```python
from build123d import *

# Parameters (mm, degrees)
SKETCH2_W           = 32
SKETCH2_H           = 30
SKETCH2_R           = 1.25
SKETCH2_R_2         = 7.25
BOSS_EXTRUDE1_DEPTH = 2
SKETCH2_4_W         = 32
SKETCH2_4_H         = 2
BOSS_EXTRUDE2_DEPTH = 35
BOSS_EXTRUDE3_DEPTH = 2
FILLET1_R           = 2
SKETCH5_W           = 7
SKETCH5_H           = 25
SKETCH5_R           = 1.6
BOSS_EXTRUDE4_DEPTH = 2
FILLET2_R           = 2
SKETCH14_W          = 16
SKETCH14_H          = 19
CUT_EXTRUDE1_DEPTH  = 52.51698749
CUT_EXTRUDE2_DEPTH  = 56.090834083
EXTRUDE_THIN1_DEPTH = 2
FILLET3_R           = 1
FILLET4_R           = 0.5
SKETCH21_R          = 1.5
CUT_EXTRUDE3_DEPTH  = 10


with BuildPart() as part:
    # Sketch2 → Boss-Extrude1 (new body)
    with BuildSketch(Plane.XY):
        Rectangle(SKETCH2_W, SKETCH2_H)
        with Locations((-8.227241336, 4.75)):
            Circle(SKETCH2_R, mode=Mode.SUBTRACT)
        with Locations((8.227241336, 4.75)):
            Circle(SKETCH2_R, mode=Mode.SUBTRACT)
        with Locations((0, -9.5)):
            Circle(SKETCH2_R, mode=Mode.SUBTRACT)
        Circle(SKETCH2_R_2, mode=Mode.SUBTRACT)
    extrude(amount=BOSS_EXTRUDE1_DEPTH)

    # Sketch2<4> → Boss-Extrude2 (add)
    with BuildSketch(Plane.XY):
        with Locations((0, -16)):
            Rectangle(SKETCH2_4_W, SKETCH2_4_H)
    extrude(amount=BOSS_EXTRUDE2_DEPTH)

    # Sketch3 → Boss-Extrude3 (add)
    with BuildSketch(Plane(origin=(16, 0, 0), x_dir=(0, 0, -1), z_dir=(1, 0, 0))):
        Polygon((-2, 6.21520857), (-22.300940927, -15), (-2, -15), align=None)
    boss_extrude3 = extrude(amount=-BOSS_EXTRUDE3_DEPTH)

    # Mirror1: Boss-Extrude3 across plane
    add(boss_extrude3.mirror(Plane.ZY))

    # Fillet1
    fillet1_edges = [part.edges().sort_by_distance(p)[0] for p in [
        (-16, 15, 1),
        (16, 15, 1),
    ]]
    fillet(fillet1_edges, radius=FILLET1_R)

    # Sketch5 → Boss-Extrude4 (add)
    # profile 1 of 2: a face of its own
    with BuildSketch(Plane(origin=(0, -15, 0), x_dir=(1, 0, 0), z_dir=(0, 1, 0))):
        with Locations((19.5, -17.5)):
            Rectangle(SKETCH5_W, SKETCH5_H)
        with Locations(Location((19.5, -26.5, 0), (0, 0, 180))):
            Circle(SKETCH5_R, mode=Mode.SUBTRACT)
        with Locations(Location((19.5, -17.5, 0), (0, 0, 180))):
            Circle(SKETCH5_R, mode=Mode.SUBTRACT)
        with Locations(Location((19.5, -8.5, 0), (0, 0, 180))):
            Circle(SKETCH5_R, mode=Mode.SUBTRACT)
    # profile 2 of 2: a face of its own
    with BuildSketch(Plane(origin=(0, -15, 0), x_dir=(1, 0, 0), z_dir=(0, 1, 0))):
        with Locations((-19.5, -17.5)):
            Rectangle(SKETCH5_W, SKETCH5_H)
        with Locations(Location((-19.5, -26.5, 0), (0, 0, 180))):
            Circle(SKETCH5_R, mode=Mode.SUBTRACT)
        with Locations(Location((-19.5, -17.5, 0), (0, 0, 180))):
            Circle(SKETCH5_R, mode=Mode.SUBTRACT)
        with Locations(Location((-19.5, -8.5, 0), (0, 0, 180))):
            Circle(SKETCH5_R, mode=Mode.SUBTRACT)
    extrude(amount=-BOSS_EXTRUDE4_DEPTH)

    # Fillet2
    fillet2_edges = [part.edges().sort_by_distance(p)[0] for p in [
        (-23, -16, 5),
        (-16, -16, 5),
        (-16, -16, 30),
        (16, -16, 35),
        (-16, -16, 35),
        (23, -16, 30),
        (16, -16, 30),
        (16, -16, 5),
        (23, -16, 5),
        (-23, -16, 30),
    ]]
    fillet(fillet2_edges, radius=FILLET2_R)

    # Sketch14 → Cut-Extrude1 (cut, through all)
    with BuildSketch(Plane(origin=(0, -15, 0), x_dir=(1, 0, 0), z_dir=(0, 1, 0))):
        with Locations((0, -19.5)):
            Rectangle(SKETCH14_W, SKETCH14_H)
    extrude(amount=-CUT_EXTRUDE1_DEPTH, mode=Mode.SUBTRACT)

    # Sketch20 → Cut-Extrude2 (cut, through all)
    with BuildSketch(Plane.ZY.offset(16)):
        Polygon((2, -12), (5, -15), (2, -15), align=None)
    extrude(amount=-CUT_EXTRUDE2_DEPTH, mode=Mode.SUBTRACT)

    # Sketch15 → Extrude-Thin1 (add)
    with BuildSketch(Plane(origin=(0, -15, 0), x_dir=(1, 0, 0), z_dir=(0, 1, 0))):
        Polygon((6.852633203, -9.033796381), (-9.147366797, -28.033796381), (-6.852633203, -29.966203619), (9.147366797, -10.966203619), align=None)
        Polygon((-9.147366797, -10.966203619), (6.852633203, -29.966203619), (9.147366797, -28.033796381), (-6.852633203, -9.033796381), align=None)
    extrude(amount=-EXTRUDE_THIN1_DEPTH)

    # Fillet3
    fillet3_edges = [part.edges().sort_by_distance(p)[0] for p in [
        (-6.03898805, -16, 10),
        (6.03898805, -16, 10),
        (-8, -16, 12.32870169),
        (-8, -16, 26.67129831),
        (6.03898805, -16, 29),
        (-6.03898805, -16, 29),
        (8, -16, 26.67129831),
        (8, -16, 12.32870169),
        (1.96101195, -16, 19.5),
        (0, -16, 21.82870169),
        (-1.96101195, -16, 19.5),
        (0, -16, 17.17129831),
    ]]
    fillet(fillet3_edges, radius=FILLET3_R)

    # Fillet4
    fillet4_edges = [part.edges().sort_by_distance(p)[0] for p in [
        (15, -12, 2),
        (15, -15, 5),
        (-15, -15, 5),
        (-15, -12, 2),
        (15, 6.21520857, 2),
        (15, -15, 22.300940927),
        (-15, 6.21520857, 2),
        (-15, -15, 22.300940927),
    ]]
    fillet(fillet4_edges, radius=FILLET4_R)

    # Sketch21 → Cut-Extrude3 (cut)
    with BuildSketch(Plane(origin=(0, 0, 0), x_dir=(-1, 0, 0), z_dir=(0, 0, -1))):
        with Locations((-8.227241336, 4.75)):
            Circle(SKETCH21_R)
        with Locations((8.227241336, 4.75)):
            Circle(SKETCH21_R)
        with Locations((0, -9.5)):
            Circle(SKETCH21_R)
    extrude(amount=-CUT_EXTRUDE3_DEPTH, mode=Mode.SUBTRACT)


solid = part.part
```
Verification items for the finished model (mm, model axes). A direction names the side the tool comes from. Coordinates: 2 decimals unless noted, no trailing zeros. Order: outer loops, then holes, each group sorted by start corner. A loop starts at its lowest first (then second) coordinate and runs counter-clockwise, first axis right, second up. Notation, with made-up numbers: (-11, 1.5) -> (43, 1.5) arc R32 ccw to (43, 33.5) -> close; hole circle Ø3 at (50.5, -24.75). An arc over 180 degrees is marked (long way). Put each result on its own line as item: value. Start each with the question number.
1) Cross-section at D-D (y = -9.5). Enter the section's corners in (x, z), plus the area to 3 significant figures.
2) Cross-section at A-A (x = -19). Enter the section's corners in (y, z).
3) Material ranges on L1, parallel to Y at x = 0, z = 0.8; L2, parallel to Z at x = -19.5, y = -15.8; L3, parallel to X at y = -2.5, z = 5.5, recorded low to high.
4) Tool access check on faces 5 (the flat face through (-20, -16, 5)), 6 (the cylindrical face through (-15.43, 14.4, 1.01)), 7 (the cylindrical face through (4.8, -16.01, 10.59)). Record the directions out of +Z, -Z, +X, -X, +Y, -Y that give a thin tool (end or side, any length) a straight path to the whole face; none if there is none.
5) Go/stop test with flat-tipped pins: pin 1 (18 mm diameter, centred on y = 0, z = 8, fed in from +X); pin 2 (4 mm diameter, centred on x = 8, z = 29.5, fed in from +Y); pin 3 (2 mm diameter, centred on x = 19.5, y = -16.5, fed in from -Z). Record where each tip stops, or that it passes through.
6) Release check for a two-part mould opening along X. For faces 1 (the cylindrical face through (20.77, -15.99, 7.53)), 2 (the cylindrical face through (0, -11, 1)), 3 (the flat face through (19, -16, 30)), 4 (the cylindrical face through (-22.43, -16.01, 29.4)) record: pulls with the +X half, pulls with the -X half, needs draft (parallel to the pull), parting line crosses it, or undercut.
7) Cross-section at B-B (y = 4.75). Enter the section's corners in (x, z).
8) Cross-section at C-C (z = 26.5). Enter the section's corners in (x, y).
Geometry check:
1. outline: (-16, 0) -> (-1.5, 0) -> (-1.5, 2) -> (-14, 2) -> (-14, 17.04) -> (-16, 17.04) -> close; (1.5, 0) -> (16, 0) -> (16, 17.04) -> (14, 17.04) -> (14, 2) -> (1.5, 2) -> close
1. area: 118 mm^2
2. outline: (-17, 5) -> (-15, 5) -> (-15, 6.98) -> (-17, 6.98) -> close; (-17, 10.02) -> (-15, 10.02) -> (-15, 15.98) -> (-17, 15.98) -> close; (-17, 19.02) -> (-15, 19.02) -> (-15, 24.98) -> (-17, 24.98) -> close; (-17, 28.02) -> (-15, 28.02) -> (-15, 30) -> (-17, 30) -> close
3. L1: y = -17 to -11, -8 to -7.25, 7.25 to 15
3. L2: z = 5 to 6.9, 10.1 to 15.9, 19.1 to 24.9, 28.1 to 30
3. L3: x = -16 to -14, 14 to 16
4. face 5: -Z, -X, +Y, -Y
4. face 6: +Z, -Z, -X, +Y
4. face 7: +Y, -Y
5. pin 1: stops at x = 16
5. pin 2: stops at y = -15
5. pin 3: stops at z = 5
6. face 1: undercut
6. face 2: undercut
6. face 3: needs draft
6. face 4: pulls with the -X half
7. outline: (-16, 0) -> (-9.73, 0) -> (-9.73, 2) -> (-14, 2) -> (-14, 3.4) -> (-16, 3.4) -> close; (-6.73, 0) -> (-5.48, 0) -> (-5.48, 2) -> (-6.73, 2) -> close; (5.48, 0) -> (6.73, 0) -> (6.73, 2) -> (5.48, 2) -> close; (9.73, 0) -> (16, 0) -> (16, 3.4) -> (14, 3.4) -> (14, 2) -> (9.73, 2) -> close
8. outline: (-23, -17) -> (-21.1, -17) -> (-21.1, -15) -> (-23, -15) -> close; (-17.9, -17) -> (-3.93, -17) -> (-3.93, -15) -> (-17.9, -15) -> close; (3.93, -17) -> (17.9, -17) -> (17.9, -15) -> (3.93, -15) -> close; (21.1, -17) -> (23, -17) -> (23, -15) -> (21.1, -15) -> close
